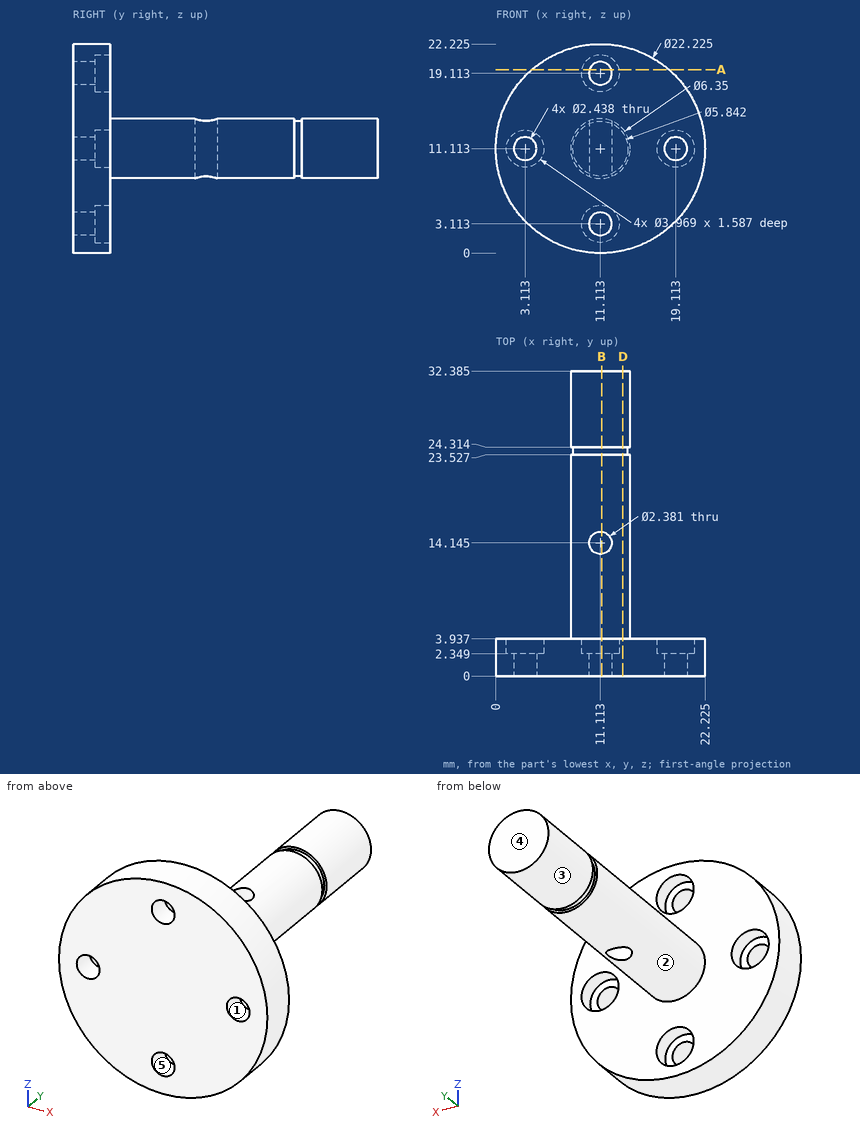
Answer from the drawing. Dimensions are ordinates in mm from the lowest x, y and z of the part. A direction names the side the tool comes from. Give positions to 0.01 mm unless a question says otherwise; leave off trailing zeros. Write each loop counter-clockwise with the first axis right and the second up, starting at its lowest first coordinate (ties: lowest second). Pieces come first, ordered by that corner, then holes. Notation, with made-up numbers: (67.25, -13.5) - (86.25, -13.5) arc R27 ccw to (86.25, 11.5) - close; hole circle Ø5 at (6, 6.25). An arc over 180 degrees is marked (long way). Answer in a Markdown table with one row per item. Add a question column.
Item 1: Flat-ended cylindrical pins translate along their axes: P1, Ø4.5, axis at x = 11.11, z = 19.11, coming from the +Y side; P2, Ø10, axis at x = 4, y = 17, coming from the +Z side; P3, Ø3, axis at y = 4.5, z = 3.5, coming from the -X side (1 decimal). Find the tip coordinate at first contact, or state that the pin passes through.
Item 2: A tool of negligible diameter and unlimited length cuts with its end or side. For the marked faces 1 and 2, from which of +Z, -Z, +X, -X, +Y, -Y can it reach the whole face along a straight path? Write none if from no direction.
Item 3: Section A-A, the plane z = 19.5 is taken. Write down the section's boundary in (x, y).
Item 4: Section B-B, the plane x = 11.25 is taken. Count the separate pieces of the cut face and the enclosed holes in it.
Item 5: Determine the mould class of the marked faces 3, 4 and 5 for opening direction Z: pulls with the +Z half, pulls with the -Z half, needs draft (parallel to the pull), parting line crosses it, or undercut.
Item 6: Section D-D, the plane x = 13.5 is taken. Write down the section's boundary in (y, z) (1 decimal), and give its area (3 significant figures).
Item 7: Find the intervals of material crossed by L1, parallel to Y at x = 7.25, z = 17.25; L2, parallel to X at y = 15, z = 9.25 (1 decimal); L3, parallel to Y at x = 10.5, z = 1.5, in increasing order.
Recorded:
| question | item | result |
|---|---|---|
| 1 | P1 | stops at y = 3.94 |
| 1 | P2 | stops at z = 13.48 |
| 1 | P3 | stops at x = 1.9 |
| 2 | face 1 | +Y, -Y |
| 2 | face 2 | +Y |
| 3 | outline | (3.82, 0) - (9.96, 0) - (9.96, 2.35) - (9.17, 2.35) - (9.17, 3.94) - (3.82, 3.94) - close; (12.27, 0) - (18.4, 0) - (18.4, 3.94) - (13.06, 3.94) - (13.06, 2.35) - (12.27, 2.35) - close |
| 4 | separate pieces | 4 |
| 4 | enclosed holes | 0 |
| 5 | face 3 | parting line crosses it |
| 5 | face 4 | needs draft |
| 5 | face 5 | undercut |
| 6 | outline | (0, 0.3) - (3.9, 0.3) - (3.9, 9) - (23.5, 9) - (23.5, 9.4) - (24.3, 9.4) - (24.3, 9) - (32.4, 9) - (32.4, 13.2) - (24.3, 13.2) - (24.3, 12.8) - (23.5, 12.8) - (23.5, 13.2) - (3.9, 13.2) - (3.9, 22) - (0, 22) - close |
| 6 | area | 204 mm2 |
| 7 | L1 | y = 0 to 3.94 |
| 7 | L2 | x = 8.5 to 10.3, 11.9 to 13.7 |
| 7 | L3 | y = 0 to 2.35 |
